Can you work these out from the model? Positions are in its coordinate system, mm. A direction names the side the tool comes from. Round coordinates to 2 decimals unless told otherwise and drop trailing zeros. Loops run counter-clockwise (first coordinate to the right, second up) from the corner with the lowest first, then second, coordinate; pieces in that order, holes last. Notation, with made-up numbers: (-21.5, 13) -> (20.5, 13) arc R17 ccw to (20.5, 46) -> close; hole circle Ø5 at (-9.75, 53). An arc over 180 degrees is marked (long way). Answer as a JSON object with one key per item and string values.
```python
from build123d import *

# Parameters (mm, degrees)
SKETCH1_W               = 29.6
SKETCH1_H               = 11
BOSS_EXTRUDE1_DEPTH     = 7
SKETCH2_W               = 6.25
SKETCH2_H               = 6.25
BOSS_EXTRUDE2_DEPTH     = 6.25
SKETCH3_W               = 7.999999319
SKETCH3_H               = 11
BOSS_EXTRUDE3_DEPTH     = 2.5
CUT_EXTRUDE1_DEPTH      = 14.25
CUT_EXTRUDE1_DEPTH_BACK = 3.5
SKETCH5_W               = 5.85
SKETCH5_H               = 10
BOSS_EXTRUDE4_DEPTH     = 8.25
CUT_EXTRUDE2_DEPTH      = 3
SKETCH7_W               = 14
SKETCH7_H               = 6.75
SKETCH7_W_2             = 6.25
SKETCH7_H_2             = 6.25
CUT_EXTRUDE3_DEPTH      = 1
FILLET1_R               = 1
FILLET2_R               = 1


with BuildPart() as part:
    # Sketch1 → Boss-Extrude1 (new body)
    with BuildSketch(Plane(origin=(0, 0, 0), x_dir=(1, 0, 0), z_dir=(0, 1, 0))):
        Rectangle(SKETCH1_W, SKETCH1_H)
    extrude(amount=BOSS_EXTRUDE1_DEPTH)

    # Sketch2 → Boss-Extrude2 (add)
    with BuildSketch(Plane(origin=(0, 7, 0), x_dir=(1, 0, 0), z_dir=(0, 1, 0))):
        Rectangle(SKETCH2_W, SKETCH2_H)
    extrude(amount=BOSS_EXTRUDE2_DEPTH)

    # Sketch3 → Boss-Extrude3 (add)
    with BuildSketch(Plane.XZ):
        with Locations((-18.79999966, 0)):
            Rectangle(SKETCH3_W, SKETCH3_H)
        Polygon((-14.8, 5.5), (-14.8, -5.5), (-11.25, -5.5), (11.25, -5.5), (14.8, -5.5), (14.8, 5.5), (11.25, 5.5), (0, 5.5), (-11.25, 5.5), align=None)
        Polygon((-9.25, 7.5), (-11.25, 5.5), (0, 5.5), (0, 7.5), align=None)
        Polygon((0, 7.5), (0, 5.5), (11.25, 5.5), (9.25, 7.5), align=None)
        with Locations((18.79999966, 0)):
            Rectangle(SKETCH3_W, SKETCH3_H)
        Polygon((11.25, -5.5), (-11.25, -5.5), (-9.25, -7.5), (0, -7.5), (9.25, -7.5), align=None)
    extrude(amount=BOSS_EXTRUDE3_DEPTH)

    # Sketch4 → Cut-Extrude1 (cut, two sides)
    with BuildSketch(Plane(origin=(0, 0, 0), x_dir=(1, 0, 0), z_dir=(0, 1, 0))) as cut_extrude1_sk:
        with BuildLine():
            Line((-18.799999319, 2), (-17.799999319, 2))
            ThreePointArc((-17.799999319, 2), (-15.799999319, 0), (-17.799999319, -2))
            Line((-17.799999319, -2), (-18.799999319, -2))
            ThreePointArc((-18.799999319, -2), (-20.799999319, 0), (-18.799999319, 2))
        make_face()
        with BuildLine():
            Line((18.799999319, 2), (17.799999319, 2))
            ThreePointArc((17.799999319, 2), (15.799999319, 0), (17.799999319, -2))
            Line((17.799999319, -2), (18.799999319, -2))
            ThreePointArc((18.799999319, -2), (20.799999319, 0), (18.799999319, 2))
        make_face()
    extrude(amount=CUT_EXTRUDE1_DEPTH, mode=Mode.SUBTRACT)
    extrude(cut_extrude1_sk.sketch, amount=-CUT_EXTRUDE1_DEPTH_BACK, mode=Mode.SUBTRACT)

    # Sketch5 → Boss-Extrude4 (add)
    with BuildSketch(Plane.XZ.offset(2.5)):
        Rectangle(SKETCH5_W, SKETCH5_H)
        with Locations((10.85, 0)):
            Rectangle(SKETCH5_W, SKETCH5_H)
        with Locations((-10.85, 0)):
            Rectangle(SKETCH5_W, SKETCH5_H)
    extrude(amount=BOSS_EXTRUDE4_DEPTH)

    # Sketch6 → Cut-Extrude2 (cut)
    with BuildSketch(Plane.XZ.offset(10.75)):
        with BuildLine():
            Line((-2, -3), (2, -3))
            ThreePointArc((2, -3), (0, -1), (-2, -3))
        make_face()
        with BuildLine():
            Line((8.85, -3), (12.85, -3))
            ThreePointArc((12.85, -3), (10.85, -1), (8.85, -3))
        make_face()
        with BuildLine():
            Line((-12.85, -3), (-8.85, -3))
            ThreePointArc((-8.85, -3), (-10.85, -1), (-12.85, -3))
        make_face()
    extrude(amount=-CUT_EXTRUDE2_DEPTH, mode=Mode.SUBTRACT)

    # Sketch7 → Cut-Extrude3 (cut)
    with BuildSketch(Plane(origin=(0, 7, 0), x_dir=(1, 0, 0), z_dir=(0, 1, 0))):
        Rectangle(SKETCH7_W, SKETCH7_H)
        Rectangle(SKETCH7_W_2, SKETCH7_H_2, mode=Mode.SUBTRACT)
    extrude(amount=-CUT_EXTRUDE3_DEPTH, mode=Mode.SUBTRACT)

    # Fillet1
    fillet1_edges = [part.edges().sort_by_distance(p)[0] for p in [
        (7, 6.5, 3.375),
        (-7, 6.5, 3.375),
        (-7, 6.5, -3.375),
        (7, 6.5, -3.375),
    ]]
    fillet(fillet1_edges, radius=FILLET1_R)

    # Fillet2
    fillet2_edges = [part.edges().sort_by_distance(p)[0] for p in [
        (3.125, 9.625, 3.125),
        (3.125, 9.625, -3.125),
        (-3.125, 9.625, -3.125),
        (-3.125, 9.625, 3.125),
    ]]
    fillet(fillet2_edges, radius=FILLET2_R)


solid = part.part
```
Q1. I want a section at C-C, the plane z = 0. Give the number of separate pieces and of enclosed holes in the cut face, then the cut area to 3 significant figures.
Determined:
{"separate pieces": "3", "enclosed holes": "0", "area": "472 mm²"}
Q2. We'd pull the mould along X, two halves only. Please class faces 6 (the flat face through (21, 0, 1)), 7 (the cylindrical face through (-20.8, -1.2, 0)), 8 (the flat face through (22.8, -1, 0)), 9 (the flat face through (-0.1, 6.5, -3.375)): pulls with the +X half, pulls with the -X half, needs draft (parallel to the pull), parting line crosses it, or undercut.
Determined:
{"face 6": "needs draft", "face 7": "undercut", "face 8": "pulls with the +X half", "face 9": "undercut"}
Q3. I want a section at D-D, the plane y = 2. Write out the boundary of the cut face in (x, z).
Determined:
{"outline": "(-14.8, -5.5) -> (14.8, -5.5) -> (14.8, 5.5) -> (-14.8, 5.5) -> close"}
Q4. I want a section at A-A, the plane y = -5.75. Write out the boundary of the cut face in (x, z) (3 decimals).
Determined:
{"outline": "(-13.775, -5) -> (-7.925, -5) -> (-7.925, 5) -> (-13.775, 5) -> close; (-2.925, -5) -> (2.925, -5) -> (2.925, 5) -> (-2.925, 5) -> close; (7.925, -5) -> (13.775, -5) -> (13.775, 5) -> (7.925, 5) -> close"}
Q5. On a 3-axis mill with a long thin cutter (end or side, diameter ignored), from which of +Z, -Z, +X, -X, +Y, -Y can I reach the whole of each face in a straight line? I mean faces 1 (the flat face through (0, 0, 7)), 2 (the flat face through (-7, 6.5, 0)), 3 (the flat face through (11, -7, 5)), 4 (the flat face through (2.925, -7, 0)), 5 (the cylindrical face through (10.9, -9.3, -1)). Say none if no direction works.
Determined:
{"face 1": "+Z, +X, -X, +Y", "face 2": "+Y", "face 3": "+Z, +X, -X, -Y", "face 4": "+Z, -Z, -Y", "face 5": "-Y"}
Q6. If I drill on L1, parallel to X at y = -5.5, z = 0.25 (3 decimals); L2, parallel to Y at x = 3, z = -1.25; L3, parallel to X at y = 0.5, z = -5, over which ranges is the centre line in solid material (lowest first)? Write a range as [from, to].
Determined:
{"L1": "[-13.775, -7.925], [-2.925, 2.925], [7.925, 13.775]", "L2": "[-2.5, 13.25]", "L3": "[-14.8, 14.8]"}
Q7. I want a section at B-B, the plane z = 4.5. Write out the boundary of the cut face in (x, y) (3 decimals).
Determined:
{"outline": "(-22.8, -2.5) -> (-13.775, -2.5) -> (-13.775, -10.75) -> (-7.925, -10.75) -> (-7.925, -2.5) -> (-2.925, -2.5) -> (-2.925, -10.75) -> (2.925, -10.75) -> (2.925, -2.5) -> (7.925, -2.5) -> (7.925, -10.75) -> (13.775, -10.75) -> (13.775, -2.5) -> (22.8, -2.5) -> (22.8, 0) -> (14.8, 0) -> (14.8, 7) -> (-14.8, 7) -> (-14.8, 0) -> (-22.8, 0) -> close"}
Q8. I'm going to push flat-ended pins straight in: pin 1 (3.5 mm diameter, centred on x = 10, y = -9.5, fed in from +Z); pin 2 (0.6 mm diameter, centred on x = 0.5, z = -2, fed in from -Y); pin 3 (0.5 mm diameter, centred on y = 6.5, z = -1, fed in from +X). Where does each tip first touch, or does it pass through?
Determined:
{"pin 1": "z = 5", "pin 2": "y = -7.75", "pin 3": "x = 14.8"}
